```python
from build123d import *

# Parameters (mm, degrees)
BOSS_EXTRUDE1_DEPTH     = 101.6
F_1_4_28_TAPPED_HOLE1_D = 5.4102


with BuildPart() as part:
    # Sketch1 → Boss-Extrude1 (new body)
    with BuildSketch(Plane(origin=(0, 0, 0), x_dir=(0, 0, -1), z_dir=(1, 0, 0))):
        Polygon((0, 19.05), (0, -19.05), (15.776765158, -19.05), (15.776765158, -17.78), (6.35, -1.452363795), (6.35, 1.452363795), (15.776765158, 17.78), (15.776765158, 19.05), align=None)
    extrude(amount=BOSS_EXTRUDE1_DEPTH)

    # 1/4-28 Tapped Hole1 (through all)
    with Locations(Plane.XY):
        with Locations((50.8, 6.35)):
            Hole(F_1_4_28_TAPPED_HOLE1_D / 2)


solid = part.part
```
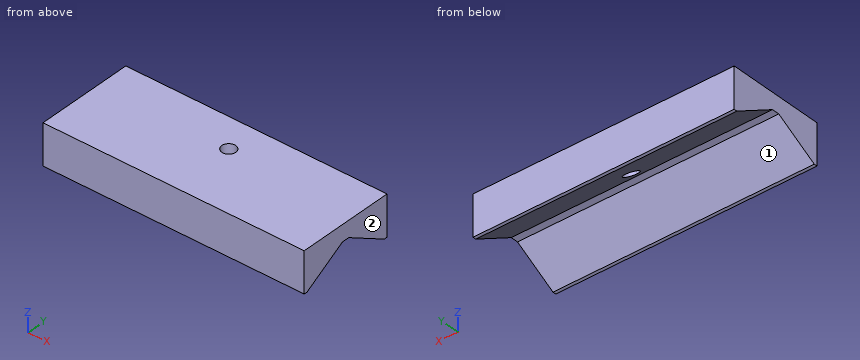
Geometry: final body of the model. Coordinates: model frame, mm. Face numbers are marked on the shaded views. A direction names the side the tool comes from. Coordinates: 2 decimals unless noted, no trailing zeros. Order: outer loops, then holes, each group sorted by start corner. A loop starts at its lowest first (then second) coordinate and runs counter-clockwise, first axis right, second up. Notation, with made-up numbers: (13.25, 86) - (33.25, 86) arc R7 ccw to (33.25, 96) - close; hole circle Ø11 at (56, -22.5). An arc over 180 degrees is marked (long way). Return JSON: item names as keys, results as strings. Group by question number.
1. Cut plane B-B (y = 6.35). Output: boundary loops of the cut face in (x, z), plus the area to 3 significant figures.
2. Set-up query: the marked faces 1 and 2. Return all of +Z, -Z, +X, -X, +Y, -Y with unobstructed straight access to the full face (end or side cutting, diameter ignored); none if empty.
3. Cut plane C-C (y = 15.5). Output: boundary loops of the cut face in (x, z).
4. Cut plane A-A (x = 56.5). Output: boundary loops of the cut face in (y, z).
5. Pin query (flat end, axial travel): pin 1 (10 mm diameter, centred on x = 66, y = -5.5, fed in from -Z); pin 2 (1.5 mm diameter, centred on x = 52, y = 5.5, fed in from +Z); pin 3 (3 mm diameter, centred on x = 39.5, y = 0, fed in from -Z). Return the tip coordinate at first contact, or that it passes through.
6. Material intervals for line 1 along Y through (x, z) = (50.8, -4); line 2 along Y through (x, z) = (50.8, -6.75); line 3 along X through (y, z) = (6.35, -3.5), sorted ascending. Write a range as [from, to].
7. Cut plane D-D (y = -9). Output: boundary loops of the cut face in (x, z).
Resolved:
{
 "1": {"outline": "(0, -9.18) - (48.09, -9.18) - (48.09, 0) - (0, 0) - close; (53.51, -9.18) - (101.6, -9.18) - (101.6, 0) - (53.51, 0) - close", "area": "883 mm²"},
 "2": {"face 1": "-Z, +X, -X", "face 2": "+Z, -Z, +X, +Y, -Y"},
 "3": {"outline": "(0, -14.46) - (101.6, -14.46) - (101.6, 0) - (0, 0) - close"},
 "4": {"outline": "(-19.05, -15.78) - (-17.78, -15.78) - (-1.45, -6.35) - (1.45, -6.35) - (17.78, -15.78) - (19.05, -15.78) - (19.05, 0) - (-19.05, 0) - close"},
 "5": {"pin 1": "stops at z = -11.57", "pin 2": "passes through", "pin 3": "stops at z = -6.38"},
 "6": {"line 1": "y = [-19.05, 3.64], [9.06, 19.05]", "line 2": "y = [-19.05, -2.15], [2.15, 3.64], [9.06, 19.05]", "line 3": "x = [0, 48.09], [53.51, 101.6]"},
 "7": {"outline": "(0, -10.71) - (101.6, -10.71) - (101.6, 0) - (0, 0) - close"}
}
